```python
from build123d import *

# Parameters (mm, degrees)
SKETCH2_R           = 4
BOSS_EXTRUDE1_DEPTH = 10
CUT_EXTRUDE1_DEPTH  = 86.791899384
SKETCH3_3_R         = 3.5
BOSS_EXTRUDE2_DEPTH = 52
SKETCH4_R           = 3.5
SKETCH4_R_2         = 6
BOSS_EXTRUDE3_DEPTH = 10
FILLET1_R           = 5


with BuildPart() as part:
    # Sketch2 → Boss-Extrude1 (new body)
    with BuildSketch(Plane(origin=(0, 0, 0), x_dir=(1, 0, 0), z_dir=(0, 1, 0))):
        Polygon((-67.5, 26), (-67.5, -4), (-35, -26), (35, -26), (67.5, -4), (67.5, 26), align=None)
        with Locations(Location((-50, 1, 0), (0, 0, 270))):
            Circle(SKETCH2_R, mode=Mode.SUBTRACT)
        with Locations(Location((50, 1, 0), (0, 0, 270))):
            Circle(SKETCH2_R, mode=Mode.SUBTRACT)
    extrude(amount=BOSS_EXTRUDE1_DEPTH)

    # Sketch3 → Cut-Extrude1 (cut, through all)
    with BuildSketch(Plane.XY.offset(26)):
        with BuildLine():
            Line((20, 0), (0, 0))
            Line((0, 0), (-20, 0))
            ThreePointArc((-20, 0), (0, -20), (20, 0))
        make_face()
        with BuildLine():
            Line((17.320508076, 10), (2.679491924, 10))
            Line((2.679491924, 10), (0, 0))
            Line((0, 0), (20, 0))
            ThreePointArc((20, 0), (19.318516526, 5.176380902), (17.320508076, 10))
        make_face()
        with BuildLine():
            Line((0, 0), (2.679491924, 10))
            Line((2.679491924, 10), (-17.320508076, 10))
            ThreePointArc((-17.320508076, 10), (-19.318516526, 5.176380902), (-20, 0))
            Line((-20, 0), (0, 0))
        make_face()
    extrude(amount=-CUT_EXTRUDE1_DEPTH, mode=Mode.SUBTRACT)


with BuildPart() as cut_extrude1_piece_1:
    # of the separate pieces the step leaves, piece 1, a body of its own (cut_extrude1_pieces)
    add(part.part.solids().sort_by_distance((67.5, 0, -26))[0])



with BuildPart() as cut_extrude1_piece_2:
    # of the separate pieces the step leaves, piece 2, a body of its own (cut_extrude1_pieces)
    add(part.part.solids().sort_by_distance((-67.5, 0, -26))[0])


with BuildPart() as cut_extrude1_piece_1_1:
    add(cut_extrude1_piece_1.part)

    add(cut_extrude1_piece_2.part)  # Boss-Extrude2 merges Cut-Extrude1 piece 2
    # Sketch3<3> → Boss-Extrude2 (add)
    with BuildSketch(Plane.XY.offset(26)):
        with BuildLine():
            ThreePointArc((-17.320508076, 10), (0, 20), (17.320508076, 10))
            Line((17.320508076, 10), (28.284271247, 10))
            ThreePointArc((28.284271247, 10), (23.442777244, 18.719941108), (16.010141687, 25.370758033))
            ThreePointArc((16.010141687, 25.370758033), (10.093942759, 37.671107225), (-1.179810402, 29.976791813))
            ThreePointArc((-1.179810402, 29.976791813), (-17.798906698, 24.149511804), (-28.284271247, 10))
            Line((-28.284271247, 10), (-17.320508076, 10))
        make_face()
        with Locations((7.764571353, 28.977774789)):
            Circle(SKETCH3_3_R, mode=Mode.SUBTRACT)
    extrude(amount=-BOSS_EXTRUDE2_DEPTH)

    # Sketch4 → Boss-Extrude3 (add)
    with BuildSketch(Plane(origin=(0, 0, -26), x_dir=(-1, 0, 0), z_dir=(0, 0, -1))):
        with BuildLine():
            ThreePointArc((62.5, 0), (62.298378138, 5.016181951), (61.694813396, 10))
            Line((61.694813396, 10), (28.284271247, 10))
            ThreePointArc((28.284271247, 10), (17.798906698, 24.149511804), (1.179810402, 29.976791813))
            ThreePointArc((1.179810402, 29.976791813), (-10.093942759, 37.671107225), (-16.010141687, 25.370758033))
            ThreePointArc((-16.010141687, 25.370758033), (-23.442777244, 18.719941108), (-28.284271247, 10))
            Line((-28.284271247, 10), (-61.694813396, 10))
            ThreePointArc((-61.694813396, 10), (-62.298378138, 5.016181951), (-62.5, 0))
            Line((-62.5, 0), (-20, 0))
            ThreePointArc((-20, 0), (0, 20), (20, 0))
            Line((20, 0), (62.5, 0))
        make_face()
        with Locations(Location((-7.764571353, 28.977774789, 0), (0, 0, 180))):
            Circle(SKETCH4_R, mode=Mode.SUBTRACT)
        with BuildLine():
            ThreePointArc((61.694813396, 10), (46.82899334, 41.391972444), (17.5, 60))
            Line((17.5, 60), (-17.5, 60))
            ThreePointArc((-17.5, 60), (-46.82899334, 41.391972444), (-61.694813396, 10))
            Line((-61.694813396, 10), (-28.284271247, 10))
            ThreePointArc((-28.284271247, 10), (-23.442777244, 18.719941108), (-16.010141687, 25.370758033))
            ThreePointArc((-16.010141687, 25.370758033), (-10.093942759, 37.671107225), (1.179810402, 29.976791813))
            ThreePointArc((1.179810402, 29.976791813), (17.798906698, 24.149511804), (28.284271247, 10))
            Line((28.284271247, 10), (61.694813396, 10))
        make_face()
        with Locations((-30.53241146, 36.387111048)):
            Circle(SKETCH4_R_2, mode=Mode.SUBTRACT)
        with Locations((30.53241146, 36.387111048)):
            Circle(SKETCH4_R_2, mode=Mode.SUBTRACT)
    extrude(amount=-BOSS_EXTRUDE3_DEPTH)

    # Fillet1
    fillet1_edges = [cut_extrude1_piece_1_1.edges().sort_by_distance(p)[0] for p in [
        (-35, 5, 26),
        (-67.5, 5, 4),
        (35, 5, 26),
        (67.5, 5, 4),
        (16.010141687, 25.370758033, 5),
        (-1.179810402, 29.976791813, 5),
    ]]
    fillet(fillet1_edges, radius=FILLET1_R)


solid = cut_extrude1_piece_1_1.part
```
Geometry check sheet. Reference: the model listing, model coordinates, mm. A direction names the side the tool comes from. Give positions to 0.01 mm unless a question says otherwise; leave off trailing zeros. Loops run counter-clockwise (first coordinate to the right, second up) from the corner with the lowest first, then second, coordinate; pieces in that order, holes last. Notation, with made-up numbers: M -18,4.5 L -1,4.5 A29 cw -1,38.5 Z; hole C 0,29.25 d6. An arc over 180 degrees is marked long. Answer as CSV lines item,"result".
Item 1: Release check for a two-part mould opening along Z. For faces 4 (the cylindrical face through (24.46, 17.37, 5.29)), 5 (the cylindrical face through (-53.549, 4.93, 0.846)), 6 (the cylindrical face through (34.953, 5.07, 25.774)) record: pulls with the +Z half, pulls with the -Z half, needs draft (parallel to the pull), parting line crosses it, or undercut.
Values:
face 4,"needs draft"
face 5,"undercut"
face 6,"pulls with the +Z half"
Item 2: Cross-section at A-A on y = 18. Record the cut outline in (x, z).
Values:
outline,"M -59.85,-26 L -8.72,-26 L -8.72,26 L -24,26 L -24,-16 L -59.85,-16 Z; M 8.72,-26 L 59.85,-26 L 59.85,-16 L 24,-16 L 24,26 L 8.72,26 Z"
Item 3: Cross-section at C-C on z = -20.5. Record the cut outline in (x, y).
Values:
outline,"M -67.5,0 L -20,0 A20 cw 20,0 L 67.5,0 L 67.5,10 L 61.69,10 A62.5 ccw 17.5,60 L -17.5,60 A62.5 ccw -61.69,10 L -67.5,10 Z; hole C -30.53,36.39 d12; hole C 7.76,28.98 d7; hole C 30.53,36.39 d12"
Item 4: Cross-section at D-D on x = -14.5. Record the cut outline in (y, z), and give its area (3 significant figures).
Values:
outline,"M 13.77,-26 L 60,-26 L 60,-16 L 26.26,-16 L 26.26,26 L 13.77,26 Z"
area,"987 mm²"
Item 5: Cross-section at B-B on x = 50. Record the cut outline in (y, z), and give its area (3 significant figures).
Values:
outline,"M 0,-26 L 37.5,-26 L 37.5,-16 L 10,-16 L 10,-5 L 0,-5 Z; M 0,3 L 10,3 L 10,15.85 L 0,15.85 Z"
area,"613 mm²"
Item 6: Access from +Z, -Z, +X, -X, +Y, -Y to the whole of each face (thin tool, end or side, straight path). Record for faces 1 (the cylindrical face through (-66.9, 5.07, 3.72)), 2 (the flat face through (0.9, 35.4, -16)), 3 (the cylindrical face through (-18.9, 23.3, 5.3)).
Values:
face 1,"+Z, -X, +Y, -Y"
face 2,"+Z, +Y"
face 3,"+Z, -X, +Y"
Item 7: Depth check by flat-ended pin: P1, Ø6.5, axis at x = 50, z = -1, coming from the -Y side; P2, Ø19, axis at x = -30.53, y = 36.39, coming from the +Z side; P3, Ø4, axis at x = -52, z = 2, coming from the +Y side; P4, Ø1.5, axis at y = 33.5, z = 19, coming from the +X side. Enter the tip coordinate at first touch or a pass-through.
Values:
P1,"passes through"
P2,"stops at z = -16"
P3,"stops at y = 10"
P4,"stops at x = 15.94"
Item 8: Material ranges on line 1 (X direction, y = 4.75, z = -1); line 2 (X direction, y = 7.25, z = -1); line 3 (Y direction, x = -10, z = -23), recorded low to high.
Values:
line 1,"x = -67.5 to -54, -46 to -19.43, 19.43 to 46, 54 to 67.5"
line 2,"x = -67.5 to -54, -46 to -18.64, 18.64 to 46, 54 to 67.5"
line 3,"y = 17.32 to 60"
